Verification items for the finished model (mm, model axes). Face numbers are marked on the shaded views. A direction names the side the tool comes from. Give positions to 0.01 mm unless a question says otherwise; leave off trailing zeros. Write each loop counter-clockwise with the first axis right and the second up, starting at its lowest first coordinate (ties: lowest second). Pieces come first, ordered by that corner, then holes. Notation, with made-up numbers: (59, 29.5) -> (90, 29.5) arc R20 ccw to (90, 46.5) -> close; hole circle Ø5 at (73, 66). An arc over 180 degrees is marked (long way). Write item = value, one per line.
from build123d import *

# Parameters (mm, degrees)
F1_R     = 6.35
F2_DEPTH = 7.9375
F3_DEPTH = 84.1375


# Not quite as in the source:
# - a variable given as a bare number and used for a length is read in inches; the dataset says mm whatever the document's units were


with BuildPart() as f2:
    # F1 (on Top) → F2 (new body)
    with BuildSketch(Plane.XY):
        Polygon((9.525, -5.499261314), (9.525, 5.499261314), (0, 10.9985226281), (-9.525, 5.499261314), (-9.525, -5.499261314), (0, -10.9985226281), align=None)
        Circle(F1_R, mode=Mode.SUBTRACT)
    extrude(amount=F2_DEPTH)

    # F1 (on Top) → F3 (join)
    with BuildSketch(Plane.XY):
        Circle(F1_R)
    extrude(amount=F3_DEPTH)


solid = f2.part
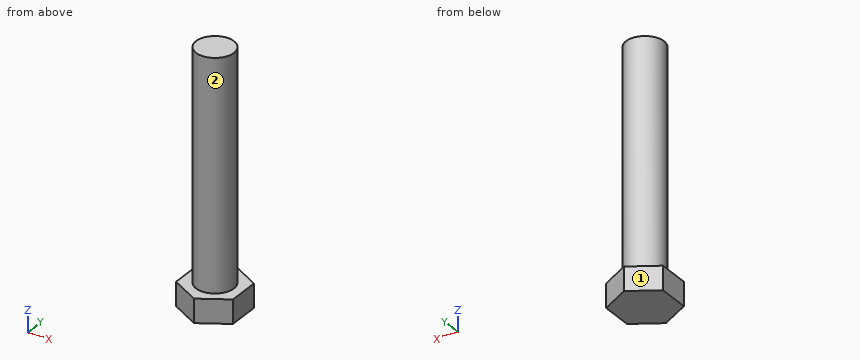
Item 1: Sectioned sample at B-B on x = 2.5. Record the cut outline in (y, z).
Response values:
outline = (-9.56, 0) -> (9.56, 0) -> (9.56, 7.94) -> (5.84, 7.94) -> (5.84, 84.14) -> (-5.84, 84.14) -> (-5.84, 7.94) -> (-9.56, 7.94) -> close
Item 2: Sectioned sample at C-C on z = 58.5. Record the cut outline in (x, y).
Response values:
outline = circle Ø12.7 at (0, 0)
Item 3: Sectioned sample at D-D on y = -9.5. Record the cut outline in (x, z).
Response values:
outline = (-2.6, 0) -> (2.6, 0) -> (2.6, 7.94) -> (-2.6, 7.94) -> close
Item 4: Material ranges on line 1 (Z direction, x = -2.25, y = 9.25); line 2 (X direction, y = -3.25, z = 19); line 3 (X direction, y = 2, z = 42.5), recorded low to high.
Response values:
line_1 = 0 to 7.94
line_2 = -5.46 to 5.46
line_3 = -6.03 to 6.03
Item 5: Go/stop test with flat-tipped pins: P1, Ø1, axis at x = -2, z = 49, coming from the -Y side; P2, Ø1.5, axis at x = 2, z = 56, coming from the +Y side; P3, Ø1.5, axis at x = -4.5, z = 35, coming from the -Y side. Record where each tip stops, or that it passes through.
Response values:
P1 = -6.17
P2 = 6.23
P3 = -5.12
Item 6: Set-up check for the marked faces 1 and 2: record each of +Z, -Z, +X, -X, +Y, -Y from which the full face is reachable in a straight line by a thin tool's end or side.
Response values:
face_1 = +Z, -Z, -X, +Y
face_2 = +Z
